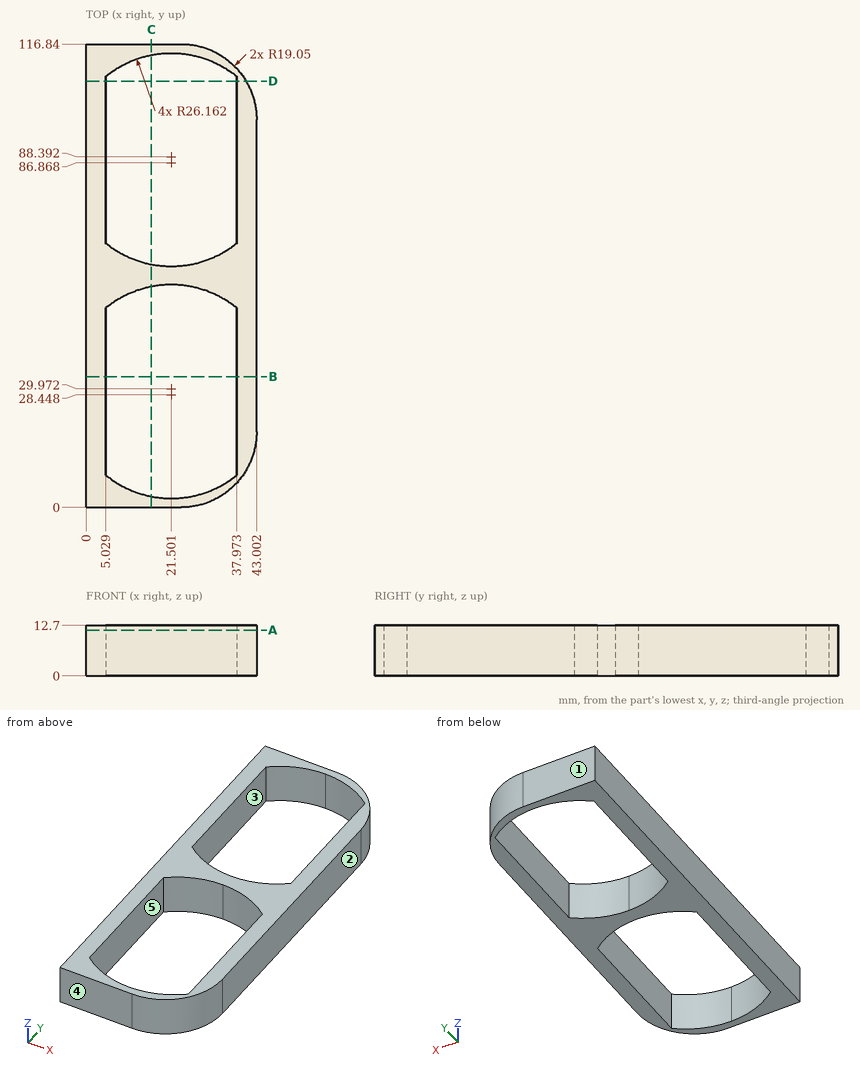
Answer from the drawing. Dimensions are ordinates in mm from the lowest x, y and z of the part. A direction names the side the tool comes from. Round coordinates to 2 decimals unless told otherwise and drop trailing zeros. Write each loop counter-clockwise with the first axis right and the second up, starting at its lowest first coordinate (ties: lowest second). Pieces come first, ordered by that corner, then holes.
1. Straight lines are drawn through the part: L1, parallel to X at y = 92, z = 2.5; L2, parallel to Y at x = 30.5, z = 4.75; L3, parallel to Y at x = 34, z = 8.75 (1 decimal). For each, find the intervals that lie inside material, in ascending order.
2. The part is cut by section A-A, the plane z = 11.5. Determine the outline of the cut face in (x, y).
3. Determine the mould class of the marked faces 1, 2 and 3 for opening direction Y: pulls with the +Y half, pulls with the -Y half, needs draft (parallel to the pull), parting line crosses it, or undercut.
4. The part is cut by section D-D, the plane y = 107.5. Determine the outline of the cut face in (x, z).
5. The part is cut by section C-C, the plane x = 16.5. Determine the outline of the cut face in (y, z).
6. Which of the six approach directions +Z, -Z, +X, -X, +Y, -Y give full straight-line access (tool end or side, diameter ignored) to the marked faces 4 and 5?
7. The part is cut by section B-B, the plane y = 33. Determine the outline of the cut face in (x, z), then the cut area to 3 significant figures.
8. Given pin 1 Ø6.5 at (y, z) = (79, 3.5) entering from -X; pin 2 Ø2 at (x, z) = (30, 7.5) entering from -Y; pin 3 Ø3 at (x, z) = (27, 10.5) entering from +Y, each flat-ended and moving along its own axis, determine where each tip first touches the part or whether it passes through.
Values:
1. L1: x = 0 to 5.03, 37.97 to 43
1. L2: y = 1.16 to 3.88, 54.54 to 62.3, 112.96 to 115.68
1. L3: y = 2.9 to 5.5, 53 to 63.9, 111.4 to 114
2. outline: (0, 0) - (23.95, 0) arc R19.05 ccw to (43, 19.05) - (43, 97.79) arc R19.05 ccw to (23.95, 116.84) - (0, 116.84) - close; hole (5.03, 8.12) arc R26.16 ccw to (37.97, 8.12) - (37.97, 50.3) arc R26.16 ccw to (5.03, 50.3) - close; hole (5.03, 66.54) arc R26.16 ccw to (37.97, 66.54) - (37.97, 108.72) arc R26.16 ccw to (5.03, 108.72) - close
3. face 1: pulls with the +Y half
3. face 2: needs draft
3. face 3: undercut
4. outline: (0, 0) - (5.03, 0) - (5.03, 12.7) - (0, 12.7) - close; (37.97, 0) - (40.34, 0) - (40.34, 12.7) - (37.97, 12.7) - close
5. outline: (0, 0) - (2.77, 0) - (2.77, 12.7) - (0, 12.7) - close; (55.65, 0) - (61.19, 0) - (61.19, 12.7) - (55.65, 12.7) - close; (114.07, 0) - (116.84, 0) - (116.84, 12.7) - (114.07, 12.7) - close
6. face 4: +Z, -Z, +X, -X, -Y
6. face 5: +Z, -Z
7. outline: (0, 0) - (5.03, 0) - (5.03, 12.7) - (0, 12.7) - close; (37.97, 0) - (43, 0) - (43, 12.7) - (37.97, 12.7) - close
7. area: 128 mm2
8. pin 1: stops at x = 0
8. pin 2: stops at y = 0.68
8. pin 3: stops at y = 116.78
